The listing builds one solid part. Answer for the finished solid, in the listing's coordinates (mm). Face numbers are marked on the shaded views. Coordinates: 2 decimals unless noted, no trailing zeros. Order: outer loops, then holes, each group sorted by start corner. A loop starts at its lowest first (then second) coordinate and runs counter-clockwise, first axis right, second up. Notation, with made-up numbers: (-2.5, -24.75) -> (53.5, -24.75) arc R19 ccw to (53.5, 9.25) -> close; hole circle Ø9 at (18.5, 63.5). An arc over 180 degrees is marked (long way). Return JSON: item names as keys, results as strings.
```python
from build123d import *

# Parameters (mm, degrees)
DIAM_TRE_DU_PER_AGE_6_0_6_1_D = 6
TROU_TARAUD_M4X0_71_D         = 3.3
TROU_TARAUD_M4X0_71_DEPTH     = 4
TROU_TARAUD_M4X0_71_TIP       = 0.991420021
D_GAGEMENT_M31_D              = 3.4


with BuildPart() as part:
    # Esquisse1 → Révolution1 (revolve)
    with BuildSketch(Plane.XY, mode=Mode.PRIVATE) as r_volution1_sk:
        Polygon((-1, 0), (1, 0), (1, 20), (-1, 20), (-1, 5), (-8, 5), (-8, 0), align=None)
    revolve(r_volution1_sk.sketch.rotate(Axis((-1031.231063335, 0, 0), (1, 0, 0)), 180), axis=Axis((-1031.231063335, 0, 0), (1, 0, 0)))

    # Diamètre du perçage Ø6.0 (6)1 (through all)
    with Locations(Plane.ZY.offset(8)):
        with Locations((0, 0)):
            Hole(DIAM_TRE_DU_PER_AGE_6_0_6_1_D / 2)

    # Trou taraudé M4x0.71
    with Locations(Plane(origin=(-4.5, 5, 0), x_dir=(0, 0, 1), z_dir=(0, 1, 0))):
        with Locations((0, 0)):
            Hole(TROU_TARAUD_M4X0_71_D / 2, depth=TROU_TARAUD_M4X0_71_DEPTH)
            with Locations((0, 0, -(TROU_TARAUD_M4X0_71_DEPTH + TROU_TARAUD_M4X0_71_TIP / 2))):  # 118° drill point
                Cone(0, TROU_TARAUD_M4X0_71_D / 2, TROU_TARAUD_M4X0_71_TIP, mode=Mode.SUBTRACT)

    # Dégagement M31 (through all)
    with Locations(Plane.ZY.offset(1)):
        with Locations((0, 15), (12.990381057, -7.5), (-12.990381057, -7.5)):
            Hole(D_GAGEMENT_M31_D / 2)


solid = part.part
```
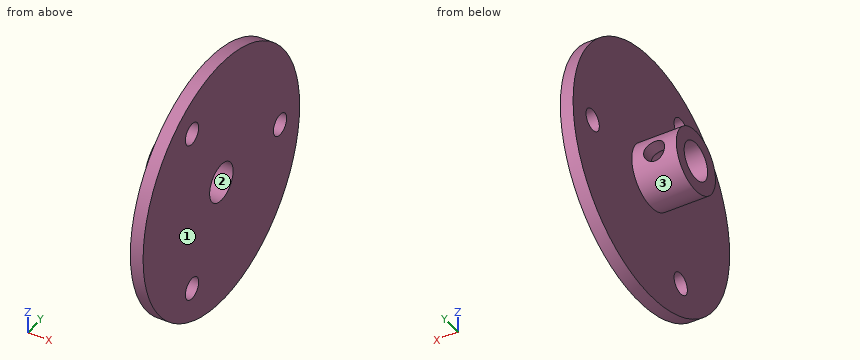
Item 1: The part is cut by section C-C on x = -0.25. Determine the outline of the cut face in (y, z), plus the area to 3 significant figures.
Answer list:
{"outline": "circle Ø40 at (0, 0); hole circle Ø3.4 at (-7.5, -12.99); hole circle Ø3.4 at (-7.5, 12.99); hole circle Ø6 at (0, 0); hole circle Ø3.4 at (15, 0)", "area": "1,200 mm2"}
Item 2: Find the intervals of material crossed by probe 1 along X at (y, z) = (3.95, 0); probe 2 along X at (y, z) = (3, 9.5); probe 3 along Y at (x, z) = (0, -0.5), in increasing order.
Answer list:
{"probe 1": "-8 to -6.15, -2.85 to 1", "probe 2": "-1 to 1", "probe 3": "-19.99 to -2.96, 2.96 to 13.38, 16.62 to 19.99"}
Item 3: Flat-ended cylindrical pins translate along their axes: pin 1 (5.5 mm diameter, centred on y = 15, z = 0, fed in from -X); pin 2 (2 mm diameter, centred on y = -7.5, z = -12.99, fed in from +X); pin 3 (2 mm diameter, centred on x = -1.5, y = -4.5, fed in from -Z). Find the tip coordinate at first contact, or state that the pin passes through.
Answer list:
{"pin 1": "x = -1", "pin 2": "through", "pin 3": "z = -19.67"}
Item 4: The part is cut by section B-B on z = 0. Determine the outline of the cut face in (x, y).
Answer list:
{"outline": "(-8, -5) -> (-1, -5) -> (-1, -20) -> (1, -20) -> (1, -3) -> (-8, -3) -> close; (-8, 3) -> (-6.15, 3) -> (-6.15, 5) -> (-8, 5) -> close; (-2.85, 3) -> (1, 3) -> (1, 13.3) -> (-1, 13.3) -> (-1, 5) -> (-2.85, 5) -> close; (-1, 16.7) -> (1, 16.7) -> (1, 20) -> (-1, 20) -> close"}
Item 5: The part is cut by section D-D on y = -6.5. Determine the outline of the cut face in (x, z).
Answer list:
{"outline": "(-1, -18.91) -> (1, -18.91) -> (1, -14.37) -> (-1, -14.37) -> close; (-1, -11.62) -> (1, -11.62) -> (1, 11.62) -> (-1, 11.62) -> close; (-1, 14.37) -> (1, 14.37) -> (1, 18.91) -> (-1, 18.91) -> close"}
Item 6: The part is cut by section A-A on y = 0. Determine the outline of the cut face in (x, z).
Answer list:
{"outline": "(-8, -5) -> (-1, -5) -> (-1, -20) -> (1, -20) -> (1, -3) -> (-8, -3) -> close; (-8, 3) -> (1, 3) -> (1, 20) -> (-1, 20) -> (-1, 5) -> (-8, 5) -> close"}
Item 7: Determine the mould class of the marked faces 1, 2 and 3 for opening direction Y: pulls with the +Y half, pulls with the -Y half, needs draft (parallel to the pull), parting line crosses it, or undercut.
Answer list:
{"face 1": "needs draft", "face 2": "undercut", "face 3": "parting line crosses it"}
